```python
from build123d import *

# Parameters (mm, degrees)
ROSCA_M10_START  = -10.35
CROQUIS1_R       = 4.25
ROSCA_M10_DEPTH  = 16
HOMBRO_D12_START = -40.35
CROQUIS2_R       = 6
HOMBRO_D12_DEPTH = 30
CABEZA_START     = -48.35
CROQUIS3_R       = 9
CABEZA_DEPTH     = 8
ALLEN_START      = -48.35
CROQUIS4_R       = 3.96
ALLEN_DEPTH      = 4.8


with BuildPart() as part:
    # Croquis1 → Rosca_M10 (new body)
    with BuildSketch(Plane(origin=(0, 0, 0), x_dir=(1, 0, 0), z_dir=(0, 1, 0)).offset(ROSCA_M10_START)):
        with Locations(Location((0, -171.45, 0), (0, 0, 270))):
            Circle(CROQUIS1_R)
    extrude(amount=ROSCA_M10_DEPTH)

    # Croquis2 → Hombro_D12 (add)
    with BuildSketch(Plane(origin=(0, 0, 0), x_dir=(1, 0, 0), z_dir=(0, 1, 0)).offset(HOMBRO_D12_START)):
        with Locations(Location((0, -171.45, 0), (0, 0, 270))):
            Circle(CROQUIS2_R)
    extrude(amount=HOMBRO_D12_DEPTH)

    # Croquis3 → Cabeza (add)
    with BuildSketch(Plane(origin=(0, 0, 0), x_dir=(1, 0, 0), z_dir=(0, 1, 0)).offset(CABEZA_START)):
        with Locations(Location((0, -171.45, 0), (0, 0, 270))):
            Circle(CROQUIS3_R)
    extrude(amount=CABEZA_DEPTH)

    # Croquis4 → Allen (cut)
    with BuildSketch(Plane(origin=(0, 0, 0), x_dir=(1, 0, 0), z_dir=(0, 1, 0)).offset(ALLEN_START)):
        with Locations(Location((0, -171.45, 0), (0, 0, 270))):
            Circle(CROQUIS4_R)
    extrude(amount=ALLEN_DEPTH, mode=Mode.SUBTRACT)


solid = part.part
```
Here's how the part is built. I have some questions about the finished solid (model axes, mm). A direction names the side the tool comes from. Coordinates: 2 decimals unless noted, no trailing zeros. Write each loop counter-clockwise with the first axis right and the second up, starting at its lowest first coordinate (ties: lowest second). Pieces come first, ordered by that corner, then holes. Notation, with made-up numbers: M 32,63 L 91,63 A23 ccw 91,73 Z; hole C 14,83 d4. An arc over 180 degrees is marked long. Answer as CSV lines item,"result". Start each with the question number.
Q1. Suppose I cut it at C-C, the plane y = 0.5. List the corners of the cut face in (x, z) for me.
Q2. Suppose I cut it at A-A, the plane z = 171.45. List the corners of the cut face in (x, y) for me, then the cut area to 3 significant figures.
Q3. Suppose I cut it at B-B, the plane x = 0. List the corners of the cut face in (y, z) for me.
Q4. For faces 1 (the cylindrical face through (0.4, -44.41, 162.46)), 2 (the cylindrical face through (0.174, -45.984, 167.494)), 3 (the flat face through (-1, -10.35, 167)), which set-ups out of +Z, -Z, +X, -X, +Y, -Y let a thin tool reach every point of the face, with its end or its side?
Q5. Will these pins go through, and if not, where does the flat tip stop? pin 1 Ø1.5 at (y, z) = (-30, 176) entering from +X; pin 2 Ø6 at (y, z) = (-5, 165) entering from +X; pin 3 Ø8 at (x, y) = (3, -20) entering from -Z.
Q6. Suppose I cut it at D-D, the plane z = 166. List the corners of the cut face in (x, y) for me.
Q7. If we mould it in two halves opening along Z, with no side actions, what happens to faces 4 (the flat face through (-4, -48.35, 173)), 5 (the cylindrical face through (1.277, -2.462, 175.504)), 6 (the flat face through (0, -43.55, 171))? For each: pulls with the +Z half, pulls with the -Z half, needs draft (parallel to the pull), parting line crosses it, or undercut.
Q8. I need wall thicknesses on probe 1 along X at (y, z) = (-44.55, 171.45); probe 2 along Y at (x, z) = (4.75, 178.75); probe 3 along Y at (x, z) = (-3.5, 166.75). Which ranges of each line are inside material? Lowest first, please. Write a range as [from, to].
Entries:
1,outline,"C 0,171.45 d8.5"
2,outline,"M -9,-48.35 L -3.96,-48.35 L -3.96,-43.55 L 3.96,-43.55 L 3.96,-48.35 L 9,-48.35 L 9,-40.35 L 6,-40.35 L 6,-10.35 L 4.25,-10.35 L 4.25,5.65 L -4.25,5.65 L -4.25,-10.35 L -6,-10.35 L -6,-40.35 L -9,-40.35 Z"
2,area,"602 mm²"
3,outline,"M -48.35,162.45 L -40.35,162.45 L -40.35,165.45 L -10.35,165.45 L -10.35,167.2 L 5.65,167.2 L 5.65,175.7 L -10.35,175.7 L -10.35,177.45 L -40.35,177.45 L -40.35,180.45 L -48.35,180.45 L -48.35,175.41 L -43.55,175.41 L -43.55,167.49 L -48.35,167.49 Z"
4,face 1,"+Y, -Y"
4,face 2,"-Y"
4,face 3,"+Y"
5,pin 1,"stops at x = 4.64"
5,pin 2,"stops at x = 2.48"
5,pin 3,"stops at z = 165.45"
6,outline,"M -7.16,-48.35 L 7.16,-48.35 L 7.16,-40.35 L 2.51,-40.35 L 2.51,-10.35 L -2.51,-10.35 L -2.51,-40.35 L -7.16,-40.35 Z"
7,face 4,"needs draft"
7,face 5,"parting line crosses it"
7,face 6,"undercut"
8,probe 1,"x = [-9, -3.96], [3.96, 9]"
8,probe 2,"y = [-48.35, -40.35]"
8,probe 3,"y = [-48.35, -10.35]"
